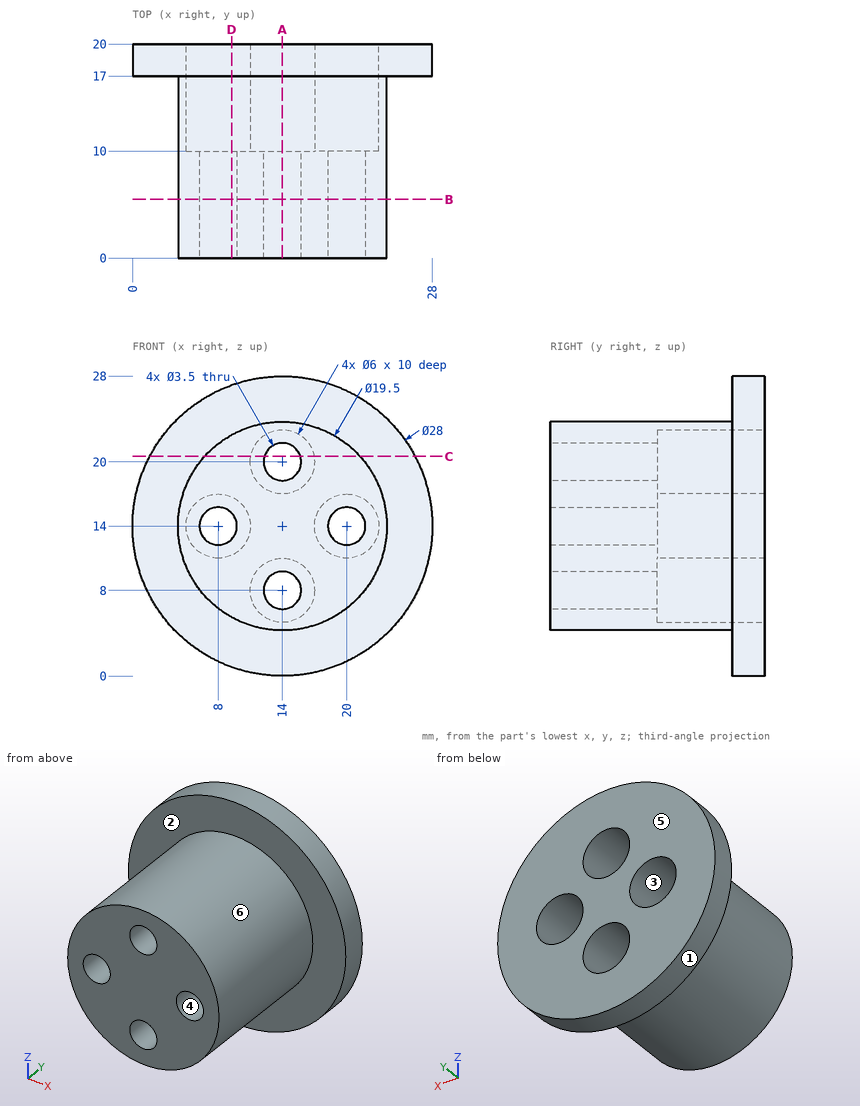
Here's the drawing with two shaded views (mm, measured from the low corner). I have some questions. A direction names the side the tool comes from. Round coordinates to 2 decimals unless told otherwise and drop trailing zeros. Loops run counter-clockwise (first coordinate to the right, second up) from the corner with the lowest first, then second, coordinate; pieces in that order, holes last. Notation, with made-up numbers: M 82,77.25 L 97,77.25 A18 cw 97,110.25 Z; hole C -12,86 d8. An arc over 180 degrees is marked long. Answer as CSV lines item,"result".
1) Which directions (+Z, -Z, +X, -X, +Y, -Y) give clear straight access to the entire face, cutting with the end or side of a thin tool? Please do the marked faces 1, 2 and 3.
From the geometry:
face 1,"+Y, -Y"
face 2,"-Y"
face 3,"+Y"
2) Imagine slicing it at C-C on z = 20.5. List the corners of the cut face in (x, y) for me, and give its area (3 significant figures).
From the geometry:
outline,"M 1.6,17 L 6.73,17 L 6.73,0 L 12.32,0 L 12.32,10 L 11.04,10 L 11.04,20 L 1.6,20 Z; M 15.68,0 L 21.27,0 L 21.27,17 L 26.4,17 L 26.4,20 L 16.96,20 L 16.96,10 L 15.68,10 Z"
area,"229 mm^2"
3) Imagine slicing it at B-B on y = 5.5. List the corners of the cut face in (x, z) for me.
From the geometry:
outline,"C 14,14 d19.5; hole C 8,14 d3.5; hole C 14,8 d3.5; hole C 14,20 d3.5; hole C 20,14 d3.5"
4) For pin 1 Ø3 at (x, z) = (8, 15) entering from +Y; pin 2 Ø5 at (x, z) = (13.5, 19) entering from +Y; pin 3 Ø3 at (x, y) = (24, 5.5) entering from -Z; pin 4 Ø1.5 at (x, z) = (23.5, 23) entering from -Y, each with a flat end and sliding along its axis, tell me the tip position at first contact or that it passes through.
From the geometry:
pin 1,"y = 10"
pin 2,"y = 20"
pin 3,"z = 9.22"
pin 4,"y = 17"
5) We'd pull the mould along Z, two halves only. Please class the marked faces 4, 5 and 6: released by +Z, released by -Z, zero draft, split by the parting line, or undercut.
From the geometry:
face 4,"undercut"
face 5,"zero draft"
face 6,"split by the parting line"
6) Imagine slicing it at D-D on x = 9.25. List the corners of the cut face in (y, z) for me, and give its area (3 significant figures).
From the geometry:
outline,"M 0,5.49 L 17,5.49 L 17,0.83 L 20,0.83 L 20,11.27 L 10,11.27 L 10,12.78 L 0,12.78 Z; M 0,15.22 L 10,15.22 L 10,16.73 L 20,16.73 L 20,27.17 L 17,27.17 L 17,22.51 L 0,22.51 Z"
area,"289 mm^2"
7) Imagine slicing it at A-A on x = 14. List the corners of the cut face in (y, z) for me, and give its area (4 significant figures).
From the geometry:
outline,"M 0,4.25 L 17,4.25 L 17,0 L 20,0 L 20,5 L 10,5 L 10,6.25 L 0,6.25 Z; M 0,9.75 L 10,9.75 L 10,11 L 20,11 L 20,17 L 10,17 L 10,18.25 L 0,18.25 Z; M 0,21.75 L 10,21.75 L 10,23 L 20,23 L 20,28 L 17,28 L 17,23.75 L 0,23.75 Z"
area,"225.5 mm^2"
8) If I drill on probe 1 along Z at (x, y) = (14, 17.5); probe 2 along Z at (x, y) = (14, 14); probe 3 along X at (y, z) = (17.75, 15.75), over which ranges is the centre line in solid material (lowest first)?
From the geometry:
probe 1,"0 to 5, 11 to 17, 23 to 28"
probe 2,"4.25 to 5, 11 to 17, 23 to 23.75"
probe 3,"0.11 to 5.56, 10.44 to 17.56, 22.44 to 27.89"
